Check sheet for the drawn part. Datum: minimum x, y, z corner. Units: mm. Give positions to 0.01 mm unless a question says otherwise; leave off trailing zeros. Loops run counter-clockwise (first coordinate to the right, second up) from the corner with the lowest first, then second, coordinate; pieces in that order, holes last. Notation, with made-up numbers: (-35.5, 32) - (-24.5, 32) arc R15 ccw to (-24.5, 52) - close; hole circle Ø1 at (73.25, 53.5). An arc over 180 degrees is marked (long way). Answer in a Markdown table with one row per item.
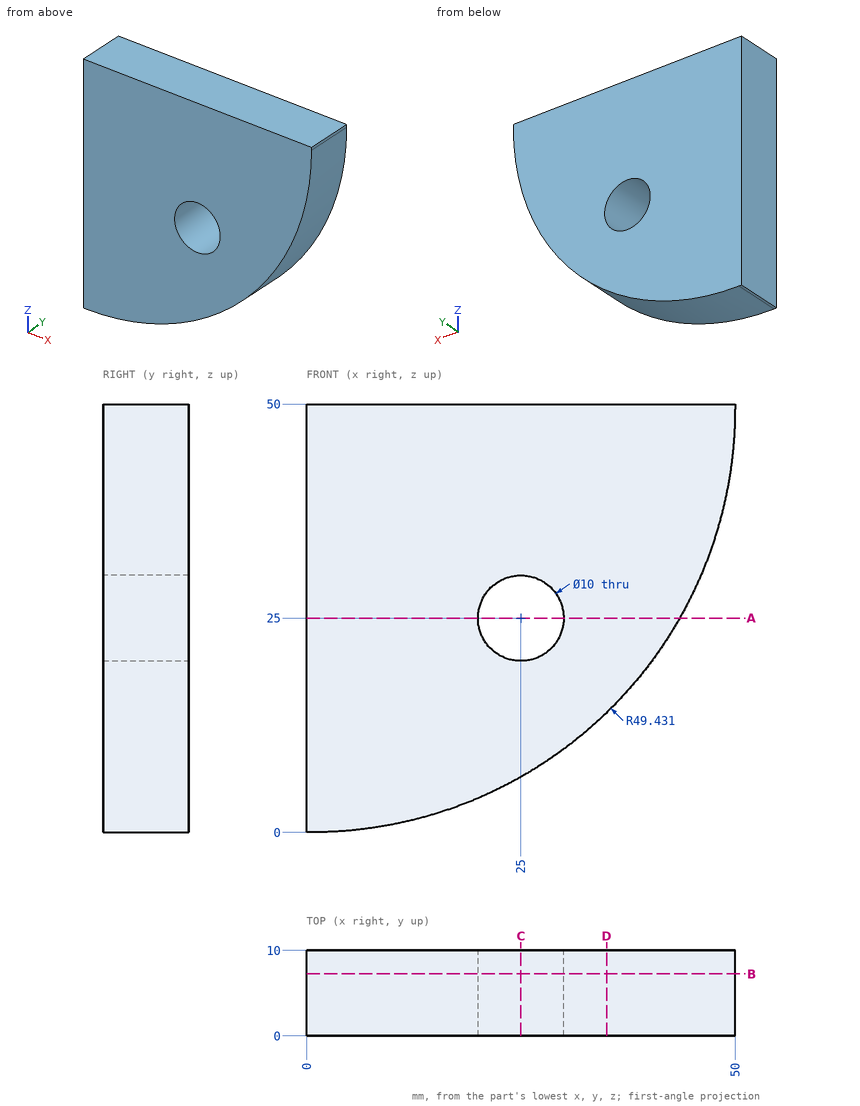
Q1. Sectioned sample at A-A (z = 25). Record the cut outline in (x, y).
Completed:
| item | result |
|---|---|
| outline | (0, 0) - (20, 0) - (20, 10) - (0, 10) - close; (30, 0) - (43.54, 0) - (43.54, 10) - (30, 10) - close |
Q2. Sectioned sample at B-B (y = 7.25). Record the cut outline in (x, z), and give its area (3 significant figures).
Completed:
| item | result |
|---|---|
| outline | (0, 0) - (0.57, 0) arc R49.43 ccw to (50, 49.43) - (50, 50) - (0, 50) - close; hole circle Ø10 at (25, 25) |
| area | 1,900 mm^2 |
Q3. Thickness scan on line 1 (Z direction, x = 29, y = 5.75) (1 decimal); line 2 (Z direction, x = 24.5, y = 5.5) (1 decimal); line 3 (X direction, y = 4.75, z = 25). Record the ranges inside material, lowest first.
Completed:
| item | result |
|---|---|
| line 1 | 9 to 22, 28 to 50 |
| line 2 | 6.2 to 20, 30 to 50 |
| line 3 | 0 to 20, 30 to 43.54 |
Q4. Sectioned sample at C-C (x = 25). Record the cut outline in (y, z), and give its area (3 significant figures).
Completed:
| item | result |
|---|---|
| outline | (0, 6.46) - (10, 6.46) - (10, 20) - (0, 20) - close; (0, 30) - (10, 30) - (10, 50) - (0, 50) - close |
| area | 335 mm^2 |
Q5. Go/stop test with a flat-tipped pin: P1, Ø1, axis at y = 5, z = 9.5, coming from the +X side. Record where the tip stops, or that it passes through.
Completed:
| item | result |
|---|---|
| P1 | x = 30.38 |
Q6. Sectioned sample at D-D (x = 35). Record the cut outline in (y, z).
Completed:
| item | result |
|---|---|
| outline | (0, 13.96) - (10, 13.96) - (10, 50) - (0, 50) - close |
